Input: part model. Units: mm. Frame: model coordinates. Give positions to 0.01 mm unless a question says otherwise; leave off trailing zeros. Loops run counter-clockwise (first coordinate to the right, second up) from the corner with the lowest first, then second, coordinate; pieces in that order, holes last. Notation, with made-up numbers: (57, -24) - (89, -24) arc R31 ccw to (89, 14) - close; hole circle Ø1 at (-20, -30). An arc over 180 degrees is marked (long way). Answer as a JSON object with one key per item and string values. Group by question number.
(1) Section query C-C (x = 4.5). Return loops of the section in (y, z).
(2) Section query B-B (z = 22.5). Return loops of the section in (x, y), plus the area to 3 significant figures.
(3) Section query A-A (x = 40.5). Return loops of the section in (y, z), plus the area to 3 significant figures.
(4) Pin query (flat end, axial travel): P1, Ø0.7, axis at y = -1, z = -32.5, coming from the +X side; P2, Ø1.4, axis at x = 50.5, y = -1.5, coming from the +Z side; P3, Ø3, axis at x = 44.5, z = 1, coming from the -Y side. Return the tip coordinate at first contact, or that it passes through.
(5) Material intervals for L1, parallel to X at y = -0.65, z = 23.5; L2, parallel to X at y = -1.6, z = 22; L3, parallel to Y at x = -5.5, z = -22.5, sorted ascending.
```python
from build123d import *

# Parameters (mm, degrees)
BOSS_EXTRUDE1_START = -16
BOSS_EXTRUDE1_DEPTH = 89.157051
SKETCH3_OUTSIDE_W   = 116.287
SKETCH3_OUTSIDE_H   = 115.611
CUT_EXTRUDE1_DEPTH  = 88.677780629
CUT_EXTRUDE2_START  = 10.52923
CUT_EXTRUDE2_DEPTH  = 98.513759981
CUT_EXTRUDE3_START  = 36.52923
CUT_EXTRUDE3_DEPTH  = 51.455299981


with BuildPart() as part:
    # Sketch2 → Boss-Extrude1 (new body)
    with BuildSketch(Plane(origin=(0, 0, 0), x_dir=(0, 0, -1), z_dir=(1, 0, 0)).offset(BOSS_EXTRUDE1_START)):
        Polygon((1.783532587, -3.008705321), (40.247767664, -2.004301248), (40.22160329, 0), (-48.232632079, 0), (-48.232632079, -1.965470246), (-6.861445597, -3.00715824), (-6.448065556, -2.007232202), (1.370510461, -2.008631392), align=None)
    extrude(amount=BOSS_EXTRUDE1_DEPTH)

    # Sketch3 outside → Cut-Extrude1 (cut, through all)
    with BuildSketch(Plane(origin=(0, 0, 0), x_dir=(1, 0, 0), z_dir=(0, 1, 0))):
        with Locations((28.5785, -3.9925)):
            Rectangle(SKETCH3_OUTSIDE_W, SKETCH3_OUTSIDE_H)
        with BuildLine():
            Line((-16, 0), (-7.992764086, -29.362208482))
            Line((-7.992764086, -29.362208482), (0.009083526, -46.765523098))
            ThreePointArc((0.009083526, -46.765523098), (2.039982857, -47.545155183), (2.868544584, -45.533721926))
            Line((2.868544584, -45.533721926), (-4.233993603, -27.882047686))
            Line((-4.233993603, -27.882047686), (-7.754483566, -11.901176784))
            Line((-7.754483566, -11.901176784), (10.497010956, -11.901176784))
            Line((10.497010956, -11.901176784), (15.258730436, -29.362208482))
            Line((15.258730436, -29.362208482), (23.274636539, -46.796099079))
            ThreePointArc((23.274636539, -46.796099079), (25.294023142, -47.545803313), (26.047958994, -45.527992762))
            Line((26.047958994, -45.527992762), (19.017500919, -30.066904431))
            Line((19.017500919, -30.066904431), (15.497010956, -11.901176784))
            Line((15.497010956, -11.901176784), (33.748505478, -11.901176784))
            Line((33.748505478, -11.901176784), (38.510224958, -29.362208482))
            Line((38.510224958, -29.362208482), (46.526131062, -46.796099079))
            ThreePointArc((46.526131062, -46.796099079), (48.545517664, -47.545803313), (49.299453516, -45.527992762))
            Line((49.299453516, -45.527992762), (42.268995441, -30.066904431))
            Line((42.268995441, -30.066904431), (38.748505478, -11.901176784))
            Line((38.748505478, -11.901176784), (57, -11.901176784))
            Line((57, -11.901176784), (61.76171948, -29.362208482))
            Line((61.76171948, -29.362208482), (69.777625584, -46.796099079))
            ThreePointArc((69.777625584, -46.796099079), (71.797012186, -47.545803313), (72.550948038, -45.527992762))
            Line((72.550948038, -45.527992762), (65.520489963, -30.066904431))
            Line((65.520489963, -30.066904431), (62, -11.901176784))
            Line((62, -11.901176784), (57.439847632, 40.22160329))
            Line((57.439847632, 40.22160329), (-8.907846133, 40.22160329))
            Line((-8.907846133, 40.22160329), (-16, 0))
        make_face(mode=Mode.SUBTRACT)
    extrude(amount=-CUT_EXTRUDE1_DEPTH, mode=Mode.SUBTRACT)

    # Sketch4 → Cut-Extrude2 (cut, through all)
    with BuildSketch(Plane(origin=(0, 0, 0), x_dir=(0, 0, -1), z_dir=(1, 0, 0)).offset(CUT_EXTRUDE2_START)):
        Polygon((24.567378522, -2.413758155), (27.144470315, 0), (40.22160329, 0), (40.247767664, -2.004301248), align=None)
    extrude(amount=-CUT_EXTRUDE2_DEPTH, mode=Mode.SUBTRACT)

    # Sketch4<2> → Cut-Extrude3 (cut, through all)
    with BuildSketch(Plane(origin=(0, 0, 0), x_dir=(0, 0, -1), z_dir=(1, 0, 0)).offset(CUT_EXTRUDE3_START)):
        Polygon((24.567378522, -2.413758155), (27.144470315, 0), (40.22160329, 0), (40.247767664, -2.004301248), align=None)
    extrude(amount=CUT_EXTRUDE3_DEPTH, mode=Mode.SUBTRACT)


solid = part.part
```
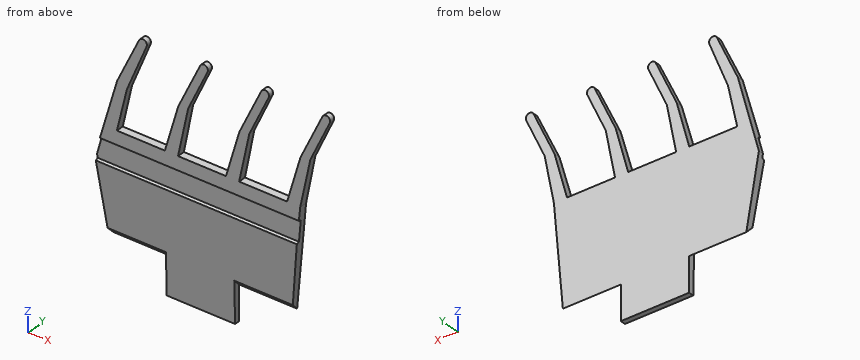
Recorded:
{
 "1": {"outline": "(-3.01, -1.78) - (-2.41, -24.57) - (0, -27.14) - (0, 11.9) - (-2.88, 11.9) - (-3.01, 6.86) - (-2.01, 6.45) - (-2.01, -1.37) - close"},
 "2": {"outline": "(-9.86, -2.61) - (-5.42, -2.61) - (-5.42, 0) - (-9.86, 0) - close; (13.39, -2.61) - (17.55, -2.61) - (17.55, 0) - (13.39, 0) - close; (36.64, -2.61) - (40.8, -2.61) - (40.8, 0) - (36.64, 0) - close; (59.89, -2.61) - (64.05, -2.61) - (64.05, 0) - (59.89, 0) - close", "area": "44.3 mm^2"},
 "3": {"outline": "(-3.01, -1.78) - (-2.41, -24.57) - (0, -27.14) - (0, 11.9) - (-2.88, 11.9) - (-3.01, 6.86) - (-2.01, 6.45) - (-2.01, -1.37) - close; (-2.65, 20.94) - (0, 20.94) - (0, 33.69) - (-2.33, 33.69) - close", "area": "129 mm^2"},
 "4": {"P1": "stops at x = 36.53", "P2": "stops at z = 11.9", "P3": "stops at y = -2.01"},
 "5": {"L1": "x = -9.59 to -5.2, 13.66 to 17.74, 36.91 to 41, 60.16 to 64.25", "L2": "x = -10 to -5.53, 13.25 to 17.45, 36.5 to 40.71, 59.75 to 63.96", "L3": "y = -2.47 to 0"}
}
